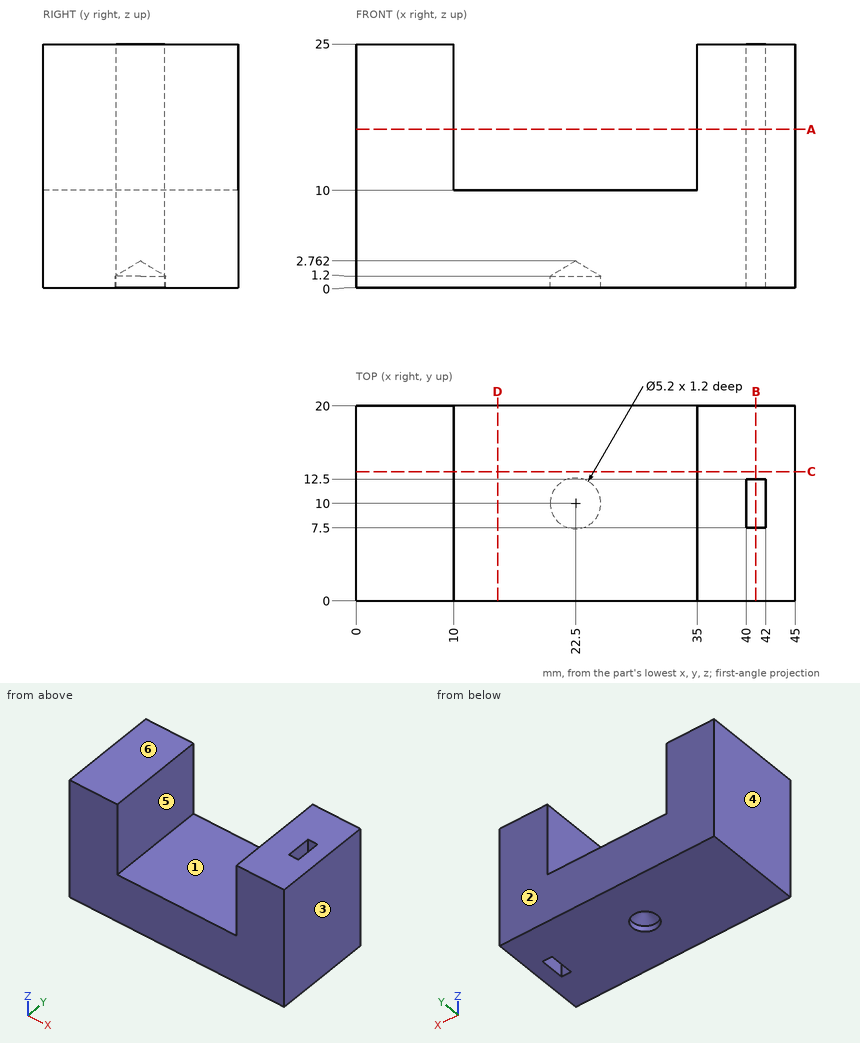
For this review, use the dimensioned drawing (mm, ordinates from the lowest corner) and the shaded views. A direction names the side the tool comes from. Coordinates: 2 decimals unless noted, no trailing zeros. Order: outer loops, then holes, each group sorted by start corner. A loop starts at its lowest first (then second) coordinate and runs counter-clockwise, first axis right, second up. Notation, with made-up numbers: (23.25, -19) - (41.25, -19) arc R12 cw to (41.25, 0) - close; hole circle Ø10 at (-37.75, 65.5). An arc over 180 degrees is marked (long way). Answer in a Markdown table with one row per item.
(1) Consider section C-C on y = 13.25. State the section outline as (x, z) points, plus the area to 3 significant figures.
Checked values:
| item | result |
|---|---|
| outline | (0, 0) - (45, 0) - (45, 25) - (35, 25) - (35, 10) - (10, 10) - (10, 25) - (0, 25) - close |
| area | 750 mm^2 |
(2) Clearance check with flat-ended pins moving along their axes: pin 1 (4 mm diameter, centred on x = 22.5, y = 10, fed in from -Z); pin 2 (5 mm diameter, centred on x = 16.5, y = 5.5, fed in from +Z). State where each tip first meets the part, or that it passes through.
Checked values:
| item | result |
|---|---|
| pin 1 | z = 1.56 |
| pin 2 | z = 10 |
(3) The part is to be moulded in two halves that separate along X. For the marked faces 3, 4, 5 and 6, say which applies: released by +X, released by -X, zero draft, split by the parting line, or undercut.
Checked values:
| item | result |
|---|---|
| face 3 | released by +X |
| face 4 | released by -X |
| face 5 | undercut |
| face 6 | zero draft |
(4) Consider section D-D on x = 14.5. State the section outline as (y, z) points.
Checked values:
| item | result |
|---|---|
| outline | (0, 0) - (20, 0) - (20, 10) - (0, 10) - close |
(5) Consider section B-B on x = 41. State the section outline as (y, z) points.
Checked values:
| item | result |
|---|---|
| outline | (0, 0) - (7.5, 0) - (7.5, 25) - (0, 25) - close; (12.5, 0) - (20, 0) - (20, 25) - (12.5, 25) - close |
(6) Consider section A-A on z = 16.25. State the section outline as (x, y) points.
Checked values:
| item | result |
|---|---|
| outline | (0, 0) - (10, 0) - (10, 20) - (0, 20) - close; (35, 0) - (45, 0) - (45, 20) - (35, 20) - close; hole (40, 7.5) - (42, 7.5) - (42, 12.5) - (40, 12.5) - close |
(7) For the marked faces 1 and 2, list the 3-axis set-ups (+Z, -Z, +X, -X, +Y, -Y) from which the entire face can be reached by the end or side of a thin tool; tool diameter is ignored.
Checked values:
| item | result |
|---|---|
| face 1 | +Z, +Y, -Y |
| face 2 | +Z, -Z, +X, -X, +Y |
(8) Wall thickness on line 1 along X through (y, z) = (11.75, 23.25); line 2 along X through (y, z) = (10, 0.9); line 3 along X through (y, z) = (9.5, 9): over which ranges is each line inside the solid? List them lowest first. Write a range as from..to.
Checked values:
| item | result |
|---|---|
| line 1 | 0..10, 35..40, 42..45 |
| line 2 | 0..19.9, 25.1..40, 42..45 |
| line 3 | 0..40, 42..45 |
